```python
from build123d import *

# Parameters (mm, degrees)
F0_W     = 0.9233176839
F0_H     = 7.9447052686
F1_DEPTH = 2


with BuildPart() as f1:
    # F0 (on Top) → F1 (new body)
    with BuildSketch(Plane.XY):
        Polygon((-6.278038602, 7.1239784385), (-6.278038602, 0), (-5.3547209181, 0), (-5.3547209181, 7.1239784385), (-2.8386367588, 7.1239784385), (-2.8386367588, 7.9447052686), (-8.7941227613, 7.9447052686), (-8.7941227613, 7.1239784385), align=None)
        with BuildLine():
            Line((-5.3547209181, 0), (-6.278038602, 0))
            Line((-6.278038602, 0), (-11.2261389214, 0))
            add(Edge.make_bspline(
                [(-11.2261389214, 0), (-11.6878851089, -0.1095461659), (-12.2509128847, -0.1095461659)],
                knots=[0.5682703015, 0.5682703015, 0.5682703015, 1, 1, 1], degree=2))
            add(Edge.make_bspline(
                [(-12.2509128847, -0.1095461659), (-13.0242578972, -0.1095461659), (-13.6025064048, 0)],
                knots=[0, 0, 0, 0.5477225575, 0.5477225575, 0.5477225575], degree=2))
            Line((-13.6025064048, 0), (-15, 0))
            Line((-15, 0), (-15, -1))
            ThreePointArc((-15, -1), (-14.7071067812, -1.7071067812), (-14, -2))
            Line((-14, -2), (-3.9937565104, -2))
            ThreePointArc((-3.9937565104, -2), (-1.8746470228, -2.8764711022), (-0.9937630208, -4.9937500136))
            Line((-0.9937630208, -4.9937500136), (-0.7549651684, -119.6167191533))
            ThreePointArc((-0.7549651684, -119.6167191533), (0.0015611574, -119.5000004874), (0.7579411203, -119.6176639074))
            Line((0.7579411203, -119.6176639074), (1.1400333331, -4.9900000556))
            ThreePointArc((1.1400333331, -4.9900000556), (2.0222347885, -2.8751470835), (4.1400166666, -2))
            Line((4.1400166666, -2), (14, -2))
            ThreePointArc((14, -2), (14.7071067812, -1.7071067812), (15, -1))
            Line((15, -1), (15, 0))
            Line((15, 0), (14.2783863676, 0))
            Line((14.2783863676, 0), (9.8495913754, 0))
            Line((9.8495913754, 0), (7.6656233698, 0))
            Line((7.6656233698, 0), (6.6118935837, 0))
            Line((6.6118935837, 0), (2.3135106938, 0))
            Line((2.3135106938, 0), (1.4597461311, 0))
            Line((1.4597461311, 0), (-0.7190053904, 0))
            Line((-0.7190053904, 0), (-1.6423230742, 0))
            Line((-1.6423230742, 0), (-5.3547209181, 0))
        make_face()
        with BuildLine():
            add(Edge.make_bspline(
                [(-11.2261389214, 0), (-11.6878851089, -0.1095461659), (-12.2509128847, -0.1095461659)],
                knots=[0.5682703015, 0.5682703015, 0.5682703015, 1, 1, 1], degree=2))
            Line((-11.2261389214, 0), (-13.6025064048, 0))
            add(Edge.make_bspline(
                [(-12.2509128847, -0.1095461659), (-13.0242578972, -0.1095461659), (-13.6025064048, 0)],
                knots=[0, 0, 0, 0.5477225575, 0.5477225575, 0.5477225575], degree=2))
        make_face()
        with BuildLine():
            Line((-13.6025064048, 0), (-11.2261389214, 0))
            add(Edge.make_bspline(
                [(-10.1860545992, 0.4781777082), (-10.6183589931, 0.1441916851), (-11.2261389214, 0)],
                knots=[0, 0, 0, 0.5682703015, 0.5682703015, 0.5682703015], degree=2))
            add(Edge.make_bspline(
                [(-9.4253173361, 2.1144148844), (-9.4253173361, 1.0659015823), (-10.1860545992, 0.4781777082)],
                knots=[0, 0, 0, 1, 1, 1], degree=2))
            add(Edge.make_bspline(
                [(-9.8948009042, 3.4394018432), (-9.4253173361, 2.9281864024), (-9.4253173361, 2.1144148844)],
                knots=[0, 0, 0, 1, 1, 1], degree=2))
            add(Edge.make_bspline(
                [(-11.6145018258, 4.3957572596), (-10.3642844723, 3.950617284), (-9.8948009042, 3.4394018432)],
                knots=[0, 0, 0, 1, 1, 1], degree=2))
            add(Edge.make_bspline(
                [(-12.7203964528, 4.881759694), (-12.3587202226, 4.6617979482), (-11.6145018258, 4.3957572596)],
                knots=[0, 0, 0, 1, 1, 1], degree=2))
            add(Edge.make_bspline(
                [(-13.2342201356, 5.3660233003), (-13.082072683, 5.1017214397), (-12.7203964528, 4.881759694)],
                knots=[0, 0, 0, 1, 1, 1], degree=2))
            add(Edge.make_bspline(
                [(-13.3863675882, 6.0424274039), (-13.3863675882, 5.6303251608), (-13.2342201356, 5.3660233003)],
                knots=[0, 0, 0, 1, 1, 1], degree=2))
            add(Edge.make_bspline(
                [(-12.9733959311, 6.917057903), (-13.3863675882, 6.6023300296), (-13.3863675882, 6.0424274039)],
                knots=[0, 0, 0, 1, 1, 1], degree=2))
            add(Edge.make_bspline(
                [(-11.8266388454, 7.2317857764), (-12.560424274, 7.2317857764), (-12.9733959311, 6.917057903)],
                knots=[0, 0, 0, 1, 1, 1], degree=2))
            add(Edge.make_bspline(
                [(-9.9139280125, 6.8196835333), (-10.8981046774, 7.2317857764), (-11.8266388454, 7.2317857764)],
                knots=[0, 0, 0, 1, 1, 1], degree=2))
            Line((-9.9139280125, 6.8196835333), (-9.6252825596, 7.6230220831))
            add(Edge.make_bspline(
                [(-11.804034081, 8.0577290906), (-10.6198921927, 8.0577290906), (-9.6252825596, 7.6230220831)],
                knots=[0, 0, 0, 1, 1, 1], degree=2))
            add(Edge.make_bspline(
                [(-13.6306729264, 7.5143453312), (-12.9412276126, 8.0577290906), (-11.804034081, 8.0577290906)],
                knots=[0, 0, 0, 1, 1, 1], degree=2))
            add(Edge.make_bspline(
                [(-14.3201182403, 6.0528603721), (-14.3201182403, 6.9709615719), (-13.6306729264, 7.5143453312)],
                knots=[0, 0, 0, 1, 1, 1], degree=2))
            add(Edge.make_bspline(
                [(-13.8445487741, 4.6348461137), (-14.3201182403, 5.1782298731), (-14.3201182403, 6.0528603721)],
                knots=[0, 0, 0, 1, 1, 1], degree=2))
            add(Edge.make_bspline(
                [(-12.2613458529, 3.6950095636), (-13.3689793079, 4.0914623544), (-13.8445487741, 4.6348461137)],
                knots=[0, 0, 0, 1, 1, 1], degree=2))
            add(Edge.make_bspline(
                [(-11.0798122066, 3.1898800209), (-11.4684402713, 3.4133194227), (-12.2613458529, 3.6950095636)],
                knots=[0, 0, 0, 1, 1, 1], degree=2))
            add(Edge.make_bspline(
                [(-10.525126065, 2.7030081725), (-10.6911841419, 2.966440619), (-11.0798122066, 3.1898800209)],
                knots=[0, 0, 0, 1, 1, 1], degree=2))
            add(Edge.make_bspline(
                [(-10.3590679882, 2.0274734829), (-10.3590679882, 2.439575726), (-10.525126065, 2.7030081725)],
                knots=[0, 0, 0, 1, 1, 1], degree=2))
            add(Edge.make_bspline(
                [(-10.8268127282, 1.0511215441), (-10.3590679882, 1.4014953921), (-10.3590679882, 2.0274734829)],
                knots=[0, 0, 0, 1, 1, 1], degree=2))
            add(Edge.make_bspline(
                [(-12.2178751521, 0.7007476961), (-11.2945574683, 0.7007476961), (-10.8268127282, 1.0511215441)],
                knots=[0, 0, 0, 1, 1, 1], degree=2))
            add(Edge.make_bspline(
                [(-13.3585463398, 0.8207268301), (-12.7829942619, 0.7007476961), (-12.2178751521, 0.7007476961)],
                knots=[0, 0, 0, 1, 1, 1], degree=2))
            add(Edge.make_bspline(
                [(-14.4244479221, 1.1458876717), (-13.9340984177, 0.9407059642), (-13.3585463398, 0.8207268301)],
                knots=[0, 0, 0, 1, 1, 1], degree=2))
            Line((-14.4244479221, 1.1458876717), (-14.4244479221, 0.2556077204))
            add(Edge.make_bspline(
                [(-13.6025064048, 0), (-14.079990402, 0.0904568546), (-14.4244479221, 0.2556077204)],
                knots=[0.5477225575, 0.5477225575, 0.5477225575, 1, 1, 1], degree=2))
        make_face()
        with Locations((-1.1806642323, 3.9723526343)):
            Rectangle(F0_W, F0_H)
        with BuildLine():
            Line((1.4597461311, 7.9447052686), (1.4597461311, 0))
            Line((1.4597461311, 0), (2.3135106938, 0))
            Line((2.3135106938, 0), (2.3135106938, 4.5157363937))
            add(Edge.make_bspline(
                [(2.2265692923, 6.6666666667), (2.3135106938, 5.4929577465), (2.3135106938, 4.5157363937)],
                knots=[0, 0, 0, 1, 1, 1], degree=2))
            Line((2.2265692923, 6.6666666667), (2.270039993, 6.6666666667))
            Line((2.270039993, 6.6666666667), (6.6118935837, 0))
            Line((6.6118935837, 0), (7.6656233698, 0))
            Line((7.6656233698, 0), (7.6656233698, 7.9447052686))
            Line((7.6656233698, 7.9447052686), (6.801425839, 7.9447052686))
            Line((6.801425839, 7.9447052686), (6.801425839, 3.3854981742))
            add(Edge.make_bspline(
                [(6.8292470875, 2.2465658146), (6.7909928708, 3.0429490523), (6.801425839, 3.3854981742)],
                knots=[0, 0, 0, 1, 1, 1], degree=2))
            add(Edge.make_bspline(
                [(6.8779342723, 1.3041210224), (6.8675013041, 1.4501825769), (6.8292470875, 2.2465658146)],
                knots=[0, 0, 0, 1, 1, 1], degree=2))
            Line((6.8779342723, 1.3041210224), (6.8344635716, 1.3041210224))
            Line((6.8344635716, 1.3041210224), (2.5030429491, 7.9447052686))
            Line((2.5030429491, 7.9447052686), (1.4597461311, 7.9447052686))
        make_face()
        Polygon((9.8495913754, 7.9447052686), (9.8495913754, 0), (14.2783863676, 0), (14.2783863676, 0.8259433142), (10.7729090593, 0.8259433142), (10.7729090593, 3.7489132325), (14.0662493479, 3.7489132325), (14.0662493479, 4.5644235785), (10.7729090593, 4.5644235785), (10.7729090593, 7.1239784385), (14.2783863676, 7.1239784385), (14.2783863676, 7.9447052686), align=None)
        with BuildLine():
            ThreePointArc((0.7579411203, -119.6176639074), (0.0015611574, -119.5000004874), (-0.7549651684, -119.6167191533))
            ThreePointArc((-0.7549651684, -119.6167191533), (-1.4769202888, -124.0171034829), (2.5, -122))
            ThreePointArc((2.5, -122), (2.0180253716, -120.5243396056), (0.7579411203, -119.6176639074))
        make_face()
    extrude(amount=F1_DEPTH)


solid = f1.part
```
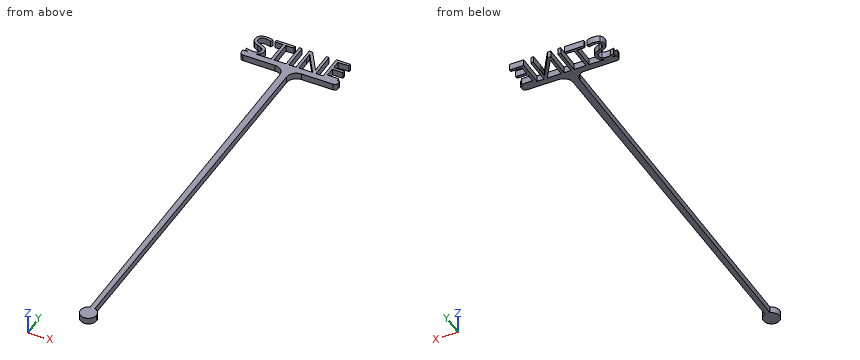
CAD build for the part. Positions are in the model's coordinates, mm. Coordinates: 2 decimals unless noted, no trailing zeros. Order: outer loops, then holes, each group sorted by start corner. A loop starts at its lowest first (then second) coordinate and runs counter-clockwise, first axis right, second up. Notation, with made-up numbers: (87, 8.25) -> (95, 8.25) arc R26 ccw to (95, 42.25) -> close; hole circle Ø1 at (69.25, 89). An arc over 180 degrees is marked (long way). Use one line per item in the form item = value. Start each with the question number.
1) Band-saw the part on A-A on y = -84. Give the cut face in (x, z).
2) Band-saw the part on B-B on y = -62.5. Give the cut face in (x, z).
3) Drill centre lines: L1, parallel to Y at x = 12.5, z = 0.45; L2, parallel to Y at x = -5, z = 1.45; L3, parallel to Y at x = -11.5, z = 1.05. Where is each one in solid material? Low to high. Write a range as [from, to].
4) Drop flat-ended pins along their axis: pin 1 (0.6 mm diameter, centred on y = 2.5, z = 1, fed in from +X); pin 2 (1 mm diameter, centred on y = -10.5, z = 0.5, fed in from +X); pin 3 (1 mm diameter, centred on y = 4.5, z = 1, fed in from -X). Give the stop position or say it passes through.
Entries:
q1.outline = (-0.83, 0) -> (0.88, 0) -> (0.88, 2) -> (-0.83, 2) -> close
q2.outline = (-0.87, 0) -> (0.95, 0) -> (0.95, 2) -> (-0.87, 2) -> close
q3.L1 = [-2, 0.83], [3.75, 4.56], [7.12, 7.94]
q3.L2 = [-2, 0], [7.12, 7.94]
q3.L3 = [-2, 0.77], [3.4, 4.35], [7.22, 8.05]
q4.pin_1 = 10.77
q4.pin_2 = 1.12
q4.pin_3 = -14.09
